```python
from build123d import *

# Parameters (mm, degrees)
CROQUIS1_R              = 7.5
SALIENTE_EXTRUIR1_DEPTH = 50
CROQUIS4_W              = 5
CROQUIS4_H              = 10
SALIENTE_EXTRUIR2_DEPTH = 12.5
CROQUIS5_R              = 2.5
CORTAR_EXTRUIR1_DEPTH   = 5
CROQUIS6_R              = 1.25
SALIENTE_EXTRUIR3_DEPTH = 10


with BuildPart() as part:
    # Croquis1 → Saliente-Extruir1 (new body)
    with BuildSketch(Plane.XY):
        Circle(CROQUIS1_R)
    extrude(amount=SALIENTE_EXTRUIR1_DEPTH)

    # Croquis4 → Saliente-Extruir2 (add)
    with BuildSketch(Plane(origin=(0, 0, 0), x_dir=(-1, 0, 0), z_dir=(0, 0, -1))):
        Rectangle(CROQUIS4_W, CROQUIS4_H)
    extrude(amount=SALIENTE_EXTRUIR2_DEPTH)

    # Croquis5 → Cortar-Extruir1 (cut)
    with BuildSketch(Plane.ZY.offset(2.5)):
        with BuildLine():
            ThreePointArc((-7.5, -5), (-11.035533906, -3.535533906), (-12.5, 0))
            Line((-12.5, 0), (-12.5, -5))
            Line((-12.5, -5), (-7.5, -5))
        make_face()
        with BuildLine():
            ThreePointArc((-12.5, 0), (-11.035533906, 3.535533906), (-7.5, 5))
            Line((-7.5, 5), (-12.5, 5))
            Line((-12.5, 5), (-12.5, 0))
        make_face()
        with Locations(Location((-7.5, 0, 0), (0, 0, 270))):
            Circle(CROQUIS5_R)
    extrude(amount=-CORTAR_EXTRUIR1_DEPTH, mode=Mode.SUBTRACT)

    # Croquis6 → Saliente-Extruir3 (add)
    with BuildSketch(Plane.XY.offset(50)):
        Circle(CROQUIS6_R)
    extrude(amount=SALIENTE_EXTRUIR3_DEPTH)

    # Croquis7 → Revolución7 (revolve)
    with BuildSketch(Plane.XY.offset(60)):
        with BuildLine():
            Line((0, 3.75), (0, -3.75))
            ThreePointArc((0, -3.75), (3.75, 0), (0, 3.75))
        make_face()
    revolve(axis=Axis((0, 7.5, 60), (0, -1, 0)))


solid = part.part
```
Geometry check sheet. Reference: the model listing, model coordinates, mm. A direction names the side the tool comes from. Give positions to 0.01 mm unless a question says otherwise; leave off trailing zeros. Order: outer loops, then holes, each group sorted by start corner. A loop starts at its lowest first (then second) coordinate and runs counter-clockwise, first axis right, second up.
1. Thickness scan on L1, parallel to Z at x = 2, y = -1; L2, parallel to X at y = 0, z = 55; L3, parallel to Z at x = -4, y = 2. Record the ranges inside material, lowest first.
2. Access from +Z, -Z, +X, -X, +Y, -Y to the whole of each face (thin tool, end or side, straight path). Record for faces 1 (the face through (-0.27, -1.22, 53.19)), 2 (the face through (0, -5, -4)), 3 (the face through (-2.5, -0.1, -4.8)), 4 (the face through (0, 5, -4)).
3. Section check D-D, the plane x = -5.25. Enter the section's corners in (y, z).
4. Section check B-B, the plane z = 21. Enter the section's corners in (x, y).
5. Section check C-C, the plane y = -6.5. Enter the section's corners in (x, z).
6. Release check for a two-part mould opening along Y. For faces 5 (the face through (-0.04, 0.54, -9.94)), 6 (the face through (2.5, -0.1, -4.8)), 7 (the face through (-7.493, 0.33, 24.65)) record: pulls with the +Y half, pulls with the -Y half, needs draft (parallel to the pull), parting line crosses it, or undercut.
7. Section check A-A, the plane x = 0. Enter the section's corners in (y, z), and give its area (3 significant figures).
8. Gauge pin test, flat ends, axial feed: pin 1 Ø3 at (x, y) = (2.5, 2.5) entering from +Z; pin 2 Ø6 at (y, z) = (-5.5, 44) entering from +X; pin 3 Ø6 at (x, z) = (5, 15.5) entering from -Y. Record the tip position at first contact, or that the pin passes through.
Values follow:
1. L1: z = -12.4 to -9.79, -5.21 to 50, 56.99 to 63.01
1. L2: x = -1.25 to 1.25
1. L3: z = 0 to 50
2. face 1: none
2. face 2: -Z, +X, -X, -Y
2. face 3: -Z, -X, +Y, -Y
2. face 4: -Z, +X, -X, +Y
3. outline: (-5.36, 0) - (5.36, 0) - (5.36, 50) - (-5.36, 50) - close
4. outline: circle Ø15 at (0, 0)
5. outline: (-3.74, 0) - (3.74, 0) - (3.74, 50) - (-3.74, 50) - close
6. face 5: undercut
6. face 6: needs draft
6. face 7: parting line crosses it
7. outline: (-7.5, 0) - (-5, 0) - (-5, -7.5) arc R5 ccw to (5, -7.5) - (5, 0) - (7.5, 0) - (7.5, 50) - (1.25, 50) - (1.25, 56.46) arc R3.75 ccw (long way) to (-1.25, 56.46) - (-1.25, 50) - (-7.5, 50) - close; hole circle Ø5 at (0, -7.5)
7. area: 905 mm2
8. pin 1: stops at z = 63.15
8. pin 2: stops at x = 7.07
8. pin 3: stops at y = -7.23
